Geometry check sheet. Reference: drawing and pictorial views, mm from the part's lowest x, y, z. Round coordinates to 2 decimals unless told otherwise and drop trailing zeros. Order: outer loops, then holes, each group sorted by start corner. A loop starts at its lowest first (then second) coordinate and runs counter-clockwise, first axis right, second up.
Q1. Cross-section at B-B on x = 1.05. Record the cut outline in (y, z), then the cut area to 3 significant figures.
Q2. Scan lines: probe 1 along Z at (x, y) = (2, 1.3); probe 2 along Y at (x, z) = (1.45, 1.5); probe 3 along X at (y, z) = (2.2, 1.25). Record each from-to range of solid material in increasing order.
Q3. Cross-section at C-C on z = 6. Record the cut outline in (x, y), then the cut area to 3 significant figures.
Q4. Depth check by flat-ended pin: P1, Ø0.5, axis at x = 1.5, z = 1, coming from the -Y side; P2, Ø0.5, axis at y = 2, z = 8.5, coming from the -X side; P3, Ø0.5, axis at y = 2.5, z = 1.5, coming from the +X side. Enter the tip coordinate at first touch or a pass-through.
Q5. Cross-section at D-D on y = 2.25. Record the cut outline in (x, z).
Q6. Cross-section at A-A on y = 1.25. Record the cut outline in (x, z), then the cut area to 3 significant figures.
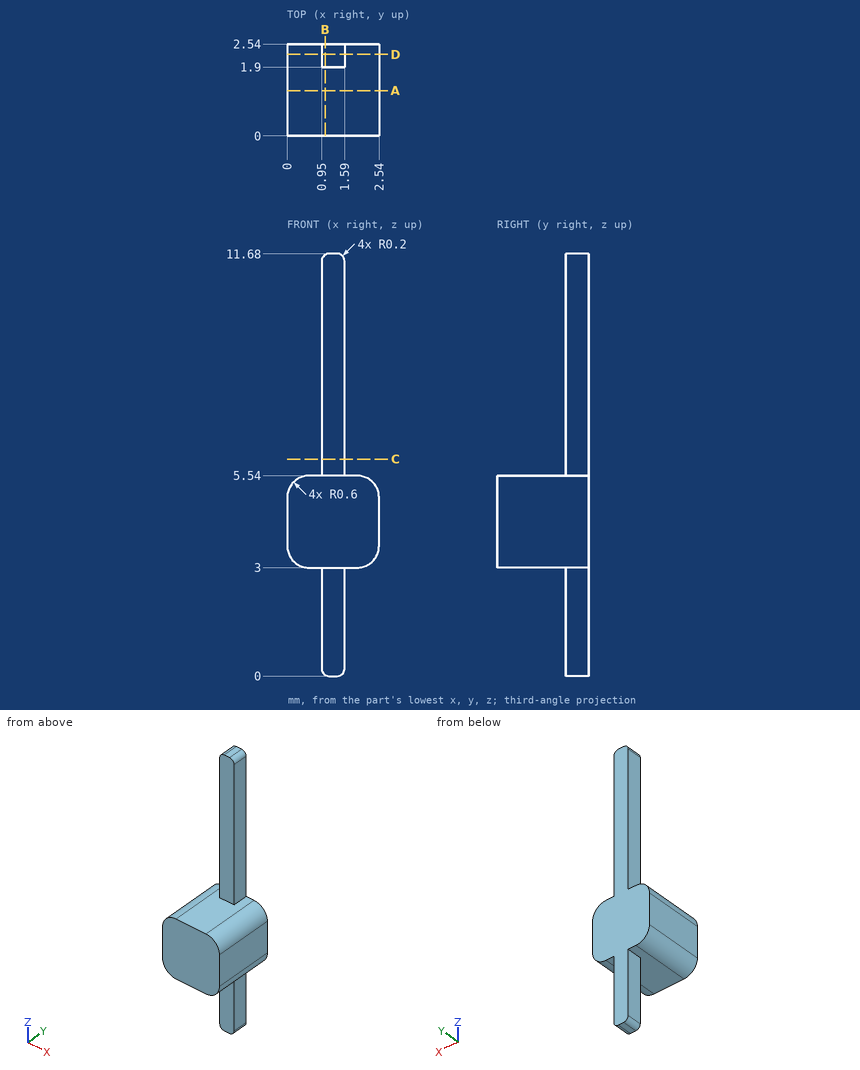
Results found:
1. outline: (0, 3) - (1.9, 3) - (1.9, 0.03) - (2.54, 0.03) - (2.54, 11.65) - (1.9, 11.65) - (1.9, 5.54) - (0, 5.54) - close
1. area: 12.3 mm2
2. probe 1: z = 3 to 5.54
2. probe 2: y = 1.9 to 2.54
2. probe 3: x = 0.95 to 1.59
3. outline: (0.95, 1.9) - (1.59, 1.9) - (1.59, 2.54) - (0.95, 2.54) - close
3. area: 0.410 mm2
4. P1: stops at y = 1.9
4. P2: stops at x = 0.95
4. P3: stops at x = 1.59
5. outline: (0, 3.6) arc R0.6 ccw to (0.6, 3) - (0.95, 3) - (0.95, 0.2) arc R0.2 ccw to (1.15, 0) - (1.39, 0) arc R0.2 ccw to (1.59, 0.2) - (1.59, 3) - (1.94, 3) arc R0.6 ccw to (2.54, 3.6) - (2.54, 4.94) arc R0.6 ccw to (1.94, 5.54) - (1.59, 5.54) - (1.59, 11.48) arc R0.2 ccw to (1.39, 11.68) - (1.15, 11.68) arc R0.2 ccw to (0.95, 11.48) - (0.95, 5.54) - (0.6, 5.54) arc R0.6 ccw to (0, 4.94) - close
6. outline: (0, 3.6) arc R0.6 ccw to (0.6, 3) - (1.94, 3) arc R0.6 ccw to (2.54, 3.6) - (2.54, 4.94) arc R0.6 ccw to (1.94, 5.54) - (0.6, 5.54) arc R0.6 ccw to (0, 4.94) - close
6. area: 6.14 mm2
